The drawing under review shows one solid part. Ordinate dimensions are in mm from its lowest x, y, z. A direction names the side the tool comes from. Coordinates: 2 decimals unless noted, no trailing zeros. Loops run counter-clockwise (first coordinate to the right, second up) from the corner with the lowest first, then second, coordinate; pieces in that order, holes last. Notation, with made-up numbers: M 84,-14.5 L 108,-14.5 A28 ccw 108,14.5 Z; hole C -37,82 d9. An arc over 180 degrees is marked long. Answer as a JSON object with one key per item and string values. Group by question number.
1. Draft analysis for pull direction Z (two halves, no side actions). For the marked faces 1, 2, 3 and 4, state which applies: +Z half, -Z half, draft (parallel to the pull), parting line (faces both ways), or undercut.
2. Insertion check: pin 1 (8 mm diameter, centred on x = 12.5, z = 10.5, fed in from -Y). The pin has a flat end and moves straight along its axis. Give the tip position at first contact, or say it passes through.
3. Consider section B-B (z = 10.25). State the section outline as (x, y) points, then the cut area to 3 significant figures.
4. Machinability: for the marked faces 5 and 6, which of the approach directions +Z, -Z, +X, -X, +Y, -Y give a long, thin tool a straight path to every point of the face, cutting with its end or side? Answer none if there is none.
5. To check wall thickness, follow probe 1 along Y at (x, z) = (18, 5.25); probe 2 along Z at (x, y) = (3.5, 88.5); probe 3 along Z at (x, y) = (4.75, 9.5). State the ranges of each line that lie inside material, in increasing order.
6. Consider section A-A (x = 6.5). State the section outline as (y, z) points.
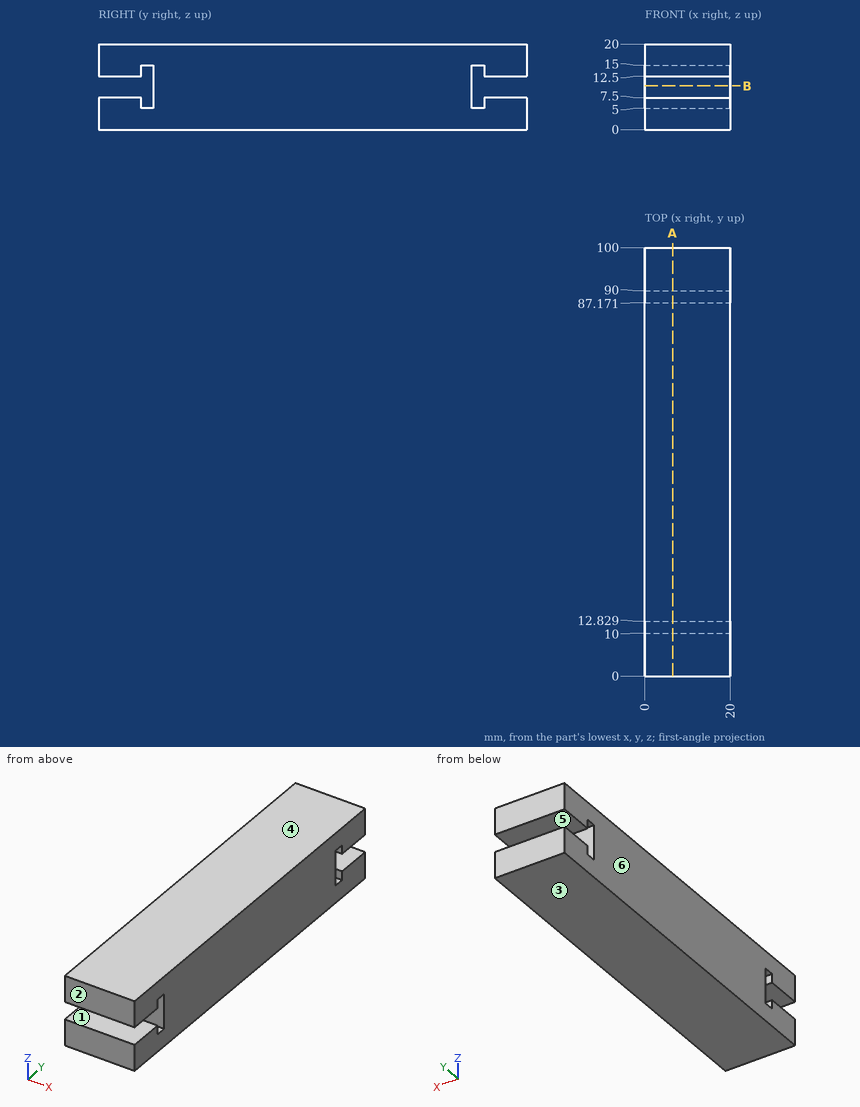
Findings below:
{
 "1": {"face 1": "undercut", "face 2": "draft", "face 3": "-Z half", "face 4": "+Z half"},
 "2": {"pin 1": "stops at y = 0"},
 "3": {"outline": "M 0,12.83 L 20,12.83 L 20,87.17 L 0,87.17 Z", "area": "1,490 mm^2"},
 "4": {"face 5": "+X, -X, +Y", "face 6": "+Z, -Z, -X, +Y, -Y"},
 "5": {"probe 1": "y = 0 to 10, 12.83 to 87.17, 90 to 100", "probe 2": "z = 0 to 5, 15 to 20", "probe 3": "z = 0 to 7.5, 12.5 to 20"},
 "6": {"outline": "M 0,0 L 100,0 L 100,7.5 L 90,7.5 L 90,5 L 87.17,5 L 87.17,15 L 90,15 L 90,12.5 L 100,12.5 L 100,20 L 0,20 L 0,12.5 L 10,12.5 L 10,15 L 12.83,15 L 12.83,5 L 10,5 L 10,7.5 L 0,7.5 Z"}
}
